The model under review builds one solid part; all positions refer to its coordinate system, in mm. A direction names the side the tool comes from. Coordinates: 2 decimals unless noted, no trailing zeros. Write each loop counter-clockwise with the first axis right and the second up, starting at its lowest first coordinate (ties: lowest second). Pieces come first, ordered by that corner, then holes. Notation, with made-up numbers: M -19.5,68.25 L 18.5,68.25 A30 ccw 18.5,92.25 Z; hole C 33.5,59.5 d10. An arc over 180 degrees is marked long. Answer as a JSON object with one key per item and string values.
```python
from build123d import *

# Parameters (mm, degrees)
SKETCH_R                = 36.83
SKETCH_R_2              = 23.622
BOSS_EXTRUDE1_DEPTH     = 6.35
SKETCH1_R               = 25.654
CUT_EXTRUDE1_DEPTH      = 4.572
F_1_4_CLEARANCE_HOLE1_D = 7.14248


with BuildPart() as part:
    # Sketch → Boss-Extrude1 (new body)
    with BuildSketch(Plane.XY):
        Circle(SKETCH_R)
        Circle(SKETCH_R_2, mode=Mode.SUBTRACT)
    extrude(amount=-BOSS_EXTRUDE1_DEPTH)

    # Sketch1 → Cut-Extrude1 (cut)
    with BuildSketch(Plane.XY):
        Circle(SKETCH1_R)
    extrude(amount=-CUT_EXTRUDE1_DEPTH, mode=Mode.SUBTRACT)

    # 1/4 Clearance Hole1 (through all)
    with Locations(Plane.XY):
        with Locations((31.75, 0), (-15.875, -27.49630657), (-15.875, 27.49630657)):
            Hole(F_1_4_CLEARANCE_HOLE1_D / 2)


solid = part.part
```
(1) For faces 5 (the face through (24.47, 7.71, -2.25)), 6 (the face through (-15.101, -30.983, -3.219)), list the 3-axis set-ups (+Z, -Z, +X, -X, +Y, -Y) from which the entire face can be reached by the end or side of a thin tool; tool diameter is ignored.
Results list:
{"face 5": "+Z", "face 6": "+Z, -Z"}
(2) Add section D-D on x = -13.5. Give the boundary of the cut face in (y, z), and give its area (3 significant figures).
Results list:
{"outline": "M -34.27,-6.35 L -30.16,-6.35 L -30.16,0 L -34.27,0 Z; M -24.83,-6.35 L -19.38,-6.35 L -19.38,-4.57 L -21.81,-4.57 L -21.81,0 L -24.83,0 Z; M 19.38,-6.35 L 24.83,-6.35 L 24.83,0 L 21.81,0 L 21.81,-4.57 L 19.38,-4.57 Z; M 30.16,-6.35 L 34.27,-6.35 L 34.27,0 L 30.16,0 Z", "area": "99.0 mm²"}
(3) For pin 1 Ø1.5 at (x, z) = (22.5, -1) entering from +Y; pin 2 Ø1 at (x, y) = (-18.5, 13.5) entering from +Z; pin 3 Ø3 at (y, z) = (-12.5, -1) entering from +X; pin 4 Ø3 at (x, z) = (20.5, -2.5) entering from +Y, all flat-tipped, find the tip position at first contact; note any pin that passes through.
Results list:
{"pin 1": "y = 29.72", "pin 2": "through", "pin 3": "x = 35.15", "pin 4": "y = 31.55"}
(4) Wall thickness on line 1 along Y through (x, z) = (0, -2.6); line 2 along X through (y, z) = (-7, -1.25); line 3 along Y through (x, z) = (9.5, -2): over which ranges is each line inside the solid? List them lowest first. Write a range as from..to.
Results list:
{"line 1": "-36.83..-25.65, 25.65..36.83", "line 2": "-36.16..-24.68, 24.68..36.16", "line 3": "-35.58..-23.83, 23.83..35.58"}
(5) Add section A-A on y = 0. Give the boundary of the cut face in (x, z).
Results list:
{"outline": "M -36.83,-6.35 L -23.62,-6.35 L -23.62,-4.57 L -25.65,-4.57 L -25.65,0 L -36.83,0 Z; M 23.62,-6.35 L 28.18,-6.35 L 28.18,0 L 25.65,0 L 25.65,-4.57 L 23.62,-4.57 Z; M 35.32,-6.35 L 36.83,-6.35 L 36.83,0 L 35.32,0 Z"}
(6) Add section C-C on y = 26.5. Give the boundary of the cut face in (x, z), and give its area (3 significant figures).
Results list:
{"outline": "M -25.58,-6.35 L -19.3,-6.35 L -19.3,0 L -25.58,0 Z; M -12.45,-6.35 L 25.58,-6.35 L 25.58,0 L -12.45,0 Z", "area": "281 mm²"}
(7) Draft analysis for pull direction X (two halves, no side actions). For faces 1 (the face through (-15.41, 31.037, -3.219)), 2 (the face through (-29.227, -22.41, -3.131)), 3 (the face through (-18.75, -14.37, -5.45)), 4 (the face through (-1, -24, -6.35)), state which applies: released by +X, released by -X, zero draft, split by the parting line, or undercut.
Results list:
{"face 1": "undercut", "face 2": "split by the parting line", "face 3": "undercut", "face 4": "zero draft"}
(8) Add section B-B on x = 0. Give the boundary of the cut face in (y, z).
Results list:
{"outline": "M -36.83,-6.35 L -23.62,-6.35 L -23.62,-4.57 L -25.65,-4.57 L -25.65,0 L -36.83,0 Z; M 23.62,-6.35 L 36.83,-6.35 L 36.83,0 L 25.65,0 L 25.65,-4.57 L 23.62,-4.57 Z"}
